```python
from build123d import *

# Parameters (mm, degrees)
F0_W          = 101.6
F0_H          = 12.7
F1_DEPTH      = 25.4
F2_W          = 10.050139
F2_H          = 23.350151
F3_DEPTH      = 127
F3_DEPTH_BACK = 127


with BuildPart() as f1:
    # F0 (on Top) → F1 (new body)
    with BuildSketch(Plane.XY):
        with Locations((-9.921525, 35.434787)):
            Rectangle(F0_W, F0_H)
    extrude(amount=F1_DEPTH)

    # F2 (on face) → F3 (cut, two sides)
    with BuildSketch(Plane(origin=(-60.721525, 0, 0), x_dir=(0, -1, 0), z_dir=(-1, 0, 0))) as f3_sk:
        with Locations((-35.486013, 12.719347)):
            Rectangle(F2_W, F2_H)
    extrude(amount=-F3_DEPTH, mode=Mode.SUBTRACT)
    extrude(f3_sk.sketch, amount=-F3_DEPTH_BACK, mode=Mode.SUBTRACT)


solid = f1.part
```
Check sheet for the modelled part. Datum: model origin and axes. Units: mm. A direction names the side the tool comes from. Give positions to 0.01 mm unless a question says otherwise; leave off trailing zeros. Order: outer loops, then holes, each group sorted by start corner. A loop starts at its lowest first (then second) coordinate and runs counter-clockwise, first axis right, second up. Notation, with made-up numbers: (12, 75.25) -> (46, 75.25) arc R16 cw to (46, 104.25) -> close; hole circle Ø8 at (50, 40.5). An arc over 180 degrees is marked (long way). Use CSV: the item, a comma, the result in double quotes. Start each with the question number.
1) Mould release check, pull along Y, two halves, no side actions. Record for faces 1 (the face through (-11, 36, 0)), 2 (the face through (-11, 36, 24.394)), 3 (the face through (-11, 41.785, 13)): released by +Y, released by -Y, zero draft, split by the parting line, or undercut.
2) Sectioned sample at A-A, the plane x = -48. Record the boundary of the cut face in (y, z), plus the area to 3 significant figures.
3) Go/stop test with a flat-tipped pin: P1, Ø5, axis at y = 36, z = 20, coming from the +X side. Record where the tip stops, or that it passes through.
4) Sectioned sample at B-B, the plane z = 19.25. Record the boundary of the cut face in (x, y), plus the area to 3 significant figures.
5) Sectioned sample at C-C, the plane y = 36. Record the boundary of the cut face in (x, z).
6) Set-up check for faces 4 (the face through (-11, 30.461, 13)), 5 (the face through (-11, 36, 25.4)): record each of +Z, -Z, +X, -X, +Y, -Y from which the full face is reachable in a straight line by a thin tool's end or side.
7) Material ranges on line 1 (Y direction, x = 25, z = 6.5); line 2 (Z direction, x = -34.5, y = 34), recorded low to high. Write a range as from..to.
Recorded:
1,face 1,"zero draft"
1,face 2,"undercut"
1,face 3,"released by +Y"
2,outline,"(29.08, 0) -> (41.78, 0) -> (41.78, 25.4) -> (29.08, 25.4) -> close; hole (30.46, 1.04) -> (40.51, 1.04) -> (40.51, 24.39) -> (30.46, 24.39) -> close"
2,area,"87.9 mm2"
3,P1,"through"
4,outline,"(-60.72, 29.08) -> (40.88, 29.08) -> (40.88, 30.46) -> (-60.72, 30.46) -> close; (-60.72, 40.51) -> (40.88, 40.51) -> (40.88, 41.78) -> (-60.72, 41.78) -> close"
4,area,"269 mm2"
5,outline,"(-60.72, 0) -> (40.88, 0) -> (40.88, 1.04) -> (-60.72, 1.04) -> close; (-60.72, 24.39) -> (40.88, 24.39) -> (40.88, 25.4) -> (-60.72, 25.4) -> close"
6,face 4,"+X, -X"
6,face 5,"+Z, +X, -X, +Y, -Y"
7,line 1,"29.08..30.46, 40.51..41.78"
7,line 2,"0..1.04, 24.39..25.4"
